from build123d import *

# Parameters (mm, degrees)
F1_DEPTH       = 1.6256
F3_DEPTH       = 17.78
F5_DEPTH       = 17.78
F6_W           = 2.54
F6_H           = 1.27
F6_W_2         = 1.27
F6_H_2         = 2.54
F7_DEPTH       = 15.24
F9_DEPTH       = 25.401
F11_DEPTH      = 25.401
F13_DEPTH      = 1.6266
F13_DEPTH_BACK = 17.781


with BuildPart() as f1:
    # F0 (on Top) → F1 (new body)
    with BuildSketch(Plane.XY):
        with BuildLine():
            Line((-15.24, -19.05), (15.24, -19.05))
            ThreePointArc((15.24, -19.05), (17.9340768363, -17.9340768363), (19.05, -15.24))
            Line((19.05, -15.24), (19.05, 15.24))
            ThreePointArc((19.05, 15.24), (17.9340768363, 17.9340768363), (15.24, 19.05))
            Line((15.24, 19.05), (-15.24, 19.05))
            ThreePointArc((-15.24, 19.05), (-17.9340768363, 17.9340768363), (-19.05, 15.24))
            Line((-19.05, 15.24), (-19.05, -15.24))
            ThreePointArc((-19.05, -15.24), (-17.9340768363, -17.9340768363), (-15.24, -19.05))
        make_face()
    extrude(amount=F1_DEPTH)

    # F2 (on face) → F3 (join)
    with BuildSketch(Plane.XY.offset(1.6256)):
        with BuildLine():
            Line((-8.89, -12.7), (8.89, -12.7))
            ThreePointArc((8.89, -12.7), (11.5840768363, -11.5840768363), (12.7, -8.89))
            Line((12.7, -8.89), (12.7, 8.89))
            ThreePointArc((12.7, 8.89), (11.5840768363, 11.5840768363), (8.89, 12.7))
            Line((8.89, 12.7), (-8.89, 12.7))
            ThreePointArc((-8.89, 12.7), (-11.5840768363, 11.5840768363), (-12.7, 8.89))
            Line((-12.7, 8.89), (-12.7, -8.89))
            ThreePointArc((-12.7, -8.89), (-11.5840768363, -11.5840768363), (-8.89, -12.7))
        make_face()
    extrude(amount=F3_DEPTH)

    # F4 (on face) → F5 (cut, through all)
    with BuildSketch(Plane.XY.offset(19.4056)):
        with BuildLine():
            ThreePointArc((-10.541, -7.493), (-9.6482614691, -9.6482614691), (-7.493, -10.541))
            Line((-7.493, -10.541), (7.493, -10.541))
            ThreePointArc((7.493, -10.541), (9.6482614691, -9.6482614691), (10.541, -7.493))
            Line((10.541, -7.493), (10.541, 7.493))
            ThreePointArc((10.541, 7.493), (9.6482614691, 9.6482614691), (7.493, 10.541))
            Line((7.493, 10.541), (-7.493, 10.541))
            ThreePointArc((-7.493, 10.541), (-9.6482614691, 9.6482614691), (-10.541, 7.493))
            Line((-10.541, 7.493), (-10.541, -7.493))
        make_face()
    extrude(amount=-F5_DEPTH, mode=Mode.SUBTRACT)

    # F6 (on face) → F7 (join)
    with BuildSketch(Plane.XY.offset(1.6256)):
        with Locations((13.97, 5.715)):
            Rectangle(F6_W, F6_H)
        with Locations((-13.97, 5.715)):
            Rectangle(F6_W, F6_H)
        with Locations((-13.97, -5.715)):
            Rectangle(F6_W, F6_H)
        with Locations((13.97, -5.715)):
            Rectangle(F6_W, F6_H)
        with Locations((5.715, 14.0176649359)):
            Rectangle(F6_W_2, F6_H_2)
        with Locations((-5.715, 14.0176649359)):
            Rectangle(F6_W_2, F6_H_2)
        with Locations((5.715, -14.0176649359)):
            Rectangle(F6_W_2, F6_H_2)
        with Locations((-5.715, -14.0176649359)):
            Rectangle(F6_W_2, F6_H_2)
    extrude(amount=F7_DEPTH)

    # F8 (on face) → F9 (cut, through all)
    with BuildSketch(Plane.XZ.offset(6.35)):
        Polygon((15.24, 16.8656), (12.7, 16.8656), (15.24, 1.6256), align=None)
        Polygon((-15.24, 1.6256), (-12.7, 16.8656), (-15.24, 16.8656), align=None)
    extrude(amount=-F9_DEPTH, mode=Mode.SUBTRACT)

    # F10 (on face) → F11 (cut, through all)
    with BuildSketch(Plane.YZ.offset(6.35)):
        Polygon((15.2876649359, 16.8656), (12.7476649359, 16.8656), (15.2876649359, 1.6256), align=None)
        Polygon((-15.2876649359, 1.6256), (-12.7476649359, 16.8656), (-15.2876649359, 16.8656), align=None)
    extrude(amount=-F11_DEPTH, mode=Mode.SUBTRACT)

    # F12 (on face) → F13 (cut, two sides)
    with BuildSketch(Plane.XY.offset(1.6256)) as f13_sk:
        with BuildLine():
            Line((15.24, 19.05), (5.6768122097, 9.268686321))
            ThreePointArc((5.6768122097, 9.268686321), (5.6969487758, 5.6969487758), (9.268686321, 5.6768122097))
            Line((9.268686321, 5.6768122097), (19.05, 15.24))
            ThreePointArc((19.05, 15.24), (17.9340768363, 17.9340768363), (15.24, 19.05))
        make_face()
    extrude(amount=-F13_DEPTH, mode=Mode.SUBTRACT)
    extrude(f13_sk.sketch, amount=F13_DEPTH_BACK, mode=Mode.SUBTRACT)


solid = f1.part
Source: CAD feature listing. Evaluate the final solid. Frame: model axes, mm. A direction names the side the tool comes from. Round coordinates to 2 decimals unless told otherwise and drop trailing zeros. Loops run counter-clockwise (first coordinate to the right, second up) from the corner with the lowest first, then second, coordinate; pieces in that order, holes last. Notation, with made-up numbers: (49.5, 13) -> (79.5, 13) arc R14 cw to (79.5, 24) -> close; hole circle Ø9 at (23, 84.5). An arc over 180 degrees is marked (long way). Answer as a JSON object with one key per item and string values. Group by question number.
Q1. Contact query for flat-ended pins moving along their axis: P1, Ø8, axis at x = 2.5, z = 12, coming from the -Y side; P2, Ø1.3, axis at y = -13.5, z = 12, coming from the +X side; P3, Ø3, axis at x = -14.5, z = 10.5, coming from the -Y side; P4, Ø0.8, axis at x = 14.5, z = 9, coming from the -Y side. Output: stop coordinate, or through.
Q2. Section query B-B (y = 3.5). Output: boundary loops of the cut face in (x, z).
Q3. Section query A-A (x = 10). Output: boundary loops of the cut face in (y, z), plus the area to 3 significant figures.
Q4. Section query D-D (z = 5.5). State how many separate pieces and enclosed holes the cut face has, plus the area to 3 significant figures.
Q5. Ray query, line 1 (X direction, y = -6.5, z = 7); line 2 (X direction, y = 13, z = 14.25). Return the intervals inside material, ascending. Write a range as from..to.
Q6. Access query for faces 1 (the cylindrical face through (-11.554, 11.614, 10.391)), 2 (the flat face through (-12.7, 0, 10)), 3 (the cylindrical face through (9.624, -9.672, 10.64)), 4 (the flat face through (12.7, 0, 10)). Directions: +Z, -Z, +X, -X, +Y, -Y. A direction counts if a zero-diameter tool reaches every point of the face in a straight line with its end or side. Return the directions, or none.
Q7. Mould query, pull axis X, two halves, no side actions, for faces 5 (the flat face through (-5.08, -13, 6)), 6 (the flat face through (13.952, 5.706, 9.352)), 7 (the flat face through (-19.05, 0, 1)). Classes: pulls with the +X half, pulls with the -X half, needs draft (parallel to the pull), parting line crosses it, or undercut.
Completed:
{
 "1": {"P1": "y = -14.07", "P2": "x = 6.35", "P3": "y = -6.35", "P4": "through"},
 "2": {"outline": "(-19.05, 0) -> (19.05, 0) -> (19.05, 1.63) -> (12.7, 1.63) -> (12.7, 19.41) -> (10.54, 19.41) -> (10.54, 1.63) -> (-10.54, 1.63) -> (-10.54, 19.41) -> (-12.7, 19.41) -> (-12.7, 1.63) -> (-19.05, 1.63) -> close"},
 "3": {"outline": "(-19.05, 0) -> (6.39, 0) -> (6.39, 1.63) -> (-9.23, 1.63) -> (-9.23, 19.41) -> (-12.53, 19.41) -> (-12.53, 1.63) -> (-19.05, 1.63) -> close; (13.69, 0) -> (19.05, 0) -> (19.05, 1.63) -> (13.69, 1.63) -> close", "area": "109 mm²"},
 "4": {"separate pieces": "5", "enclosed holes": "0", "area": "201 mm²"},
 "5": {"line 1": "-12.7..-10.54, 10.54..12.7", "line 2": "-6.35..-5.08, 5.08..6.35"},
 "6": {"face 1": "+Z, -X, +Y", "face 2": "+Z, -X", "face 3": "+Z", "face 4": "+Z, +X"},
 "7": {"face 5": "undercut", "face 6": "pulls with the +X half", "face 7": "pulls with the -X half"}
}
